Model file for the job. Use its own axes, mm. A direction names the side the tool comes from. Round coordinates to 2 decimals unless told otherwise and drop trailing zeros. Loops run counter-clockwise (first coordinate to the right, second up) from the corner with the lowest first, then second, coordinate; pieces in that order, holes last. Notation, with made-up numbers: (8, 19.25) -> (61, 19.25) arc R13 ccw to (61, 36.25) -> close; hole circle Ø11 at (69.25, -11). An arc over 180 degrees is marked (long way). Use a Markdown table: item, result.
from build123d import *

# Parameters (mm, degrees)
F1_DEPTH = 63.5
F0_W     = 25.4
F0_H     = 19.05
F2_DEPTH = 25.4
F3_DEPTH = 7.9375


with BuildPart() as f1:
    # F0 (on Front) → F1 (new body, symmetric)
    with BuildSketch(Plane.XZ):
        Polygon((41.275, -9.525), (41.275, 9.525), (22.225, 9.525), (-41.275, 9.525), (-41.275, -9.525), align=None)
    extrude(amount=F1_DEPTH, both=True)

    # F0 (on Front) → F2 (join, symmetric)
    with BuildSketch(Plane.XZ):
        with BuildLine():
            Line((22.225, 9.525), (41.275, 9.525))
            Line((41.275, 9.525), (41.275, 27.0002))
            ThreePointArc((41.275, 27.0002), (45.9246798487, 38.2255201513), (57.15, 42.8752))
            Line((57.15, 42.8752), (60.325, 42.8752))
            Line((60.325, 42.8752), (60.325, 61.9252))
            Line((60.325, 61.9252), (57.15, 61.9252))
            add(Edge.make_bspline(
                [(55.6374674655, 61.8924322349), (56.1423918101, 61.9048336292), (56.6465953403, 61.9157496607), (57.15, 61.9252)],
                knots=[110.2644548884, 110.2644548884, 110.2644548884, 110.2644548884, 111.5045361635, 111.5045361635, 111.5045361635, 111.5045361635], degree=3))
            ThreePointArc((55.6374674655, 61.8924322349), (31.9252024412, 51.1552245936), (22.225, 27.0002))
            Line((22.225, 27.0002), (22.225, 9.525))
        make_face()
        with Locations((73.025, 52.4002)):
            Rectangle(F0_W, F0_H)
    extrude(amount=F2_DEPTH, both=True)

    # F0 (on Front) → F3 (join, symmetric)
    with BuildSketch(Plane.XZ):
        with BuildLine():
            Line((-41.275, 9.525), (22.225, 9.525))
            Line((22.225, 9.525), (22.225, 27.0002))
            ThreePointArc((22.225, 27.0002), (31.9252024412, 51.1552245936), (55.6374674655, 61.8924322349))
            add(Edge.make_bspline(
                [(-41.275, 9.525), (-39.8543103668, 47.9433842004), (10.7410491974, 60.789735975), (55.6374674655, 61.8924322349)],
                knots=[0, 0, 0, 0, 110.2644548884, 110.2644548884, 110.2644548884, 110.2644548884], degree=3))
        make_face()
    extrude(amount=F3_DEPTH, both=True)

    # F0 (on Front) → F4 (revolve)
    with BuildSketch(Plane.XZ):
        Polygon((85.725, 61.9252), (85.725, 42.8752), (85.725, 38.1), (111.125, 38.1), (111.125, 66.675), (85.725, 66.675), align=None)
    revolve(axis=Axis((85.725, 0, 52.3875), (0, 0, 1)))


solid = f1.part
Q1. Drill centre lines: L1, parallel to Z at x = 17, y = -20 (3 decimals); L2, parallel to Y at x = -11, z = 38; L3, parallel to Y at x = 77.5, z = 48.5. Where is each one in solid material? Low to high. Write a range as from..to.
Results list:
| item | result |
|---|---|
| L1 | z = -9.525..9.525 |
| L2 | y = -7.94..7.94 |
| L3 | y = -25.4..25.4 |
Q2. Flat gauge pins, fed straight in: pin 1 (16.5 mm diameter, centred on x = 2.5, y = -47.5, fed in from +Z) (3 decimals); pin 2 (5 mm diameter, centred on y = 19.5, z = 54.5, fed in from +X); pin 3 (11 mm diameter, centred on y = -10, z = 3, fed in from +X) (3 decimals). Where does each tip first touch, or does it go through?
Results list:
| item | result |
|---|---|
| pin 1 | stops at z = 9.525 |
| pin 2 | stops at x = 104.6 |
| pin 3 | stops at x = 41.275 |
Q3. Band-saw the part on A-A, the plane y = -29. Give the cut face in (x, z) (3 decimals).
Results list:
| item | result |
|---|---|
| outline | (-41.275, -9.525) -> (41.275, -9.525) -> (41.275, 9.525) -> (-41.275, 9.525) -> close |
Q4. Pull direction X, two halves, no side cores. Call faces 1 (the face through (60, 2, 42.875)), 2 (the face through (60, -2, 61.925)), 3 (the face through (32.18, 16.55, 51.42)): released by +X, released by -X, zero draft, split by the parting line, or undercut.
Results list:
| item | result |
|---|---|
| face 1 | undercut |
| face 2 | zero draft |
| face 3 | released by -X |
Q5. Tool access for faces 4 (the face through (46, 25.4, 42)), 5 (the face through (45.8, -0.4, 38.1)), 6 (the face through (-4, 7.938, 30)), 7 (the face through (-4, -7.938, 30)), 8 (the face through (41.275, -1, 4)): list every direction of +Z, -Z, +X, -X, +Y, -Y with a clear straight run to the whole face (end or side of a thin tool).
Results list:
| item | result |
|---|---|
| face 4 | +Z, +X, -X, +Y |
| face 5 | -Z, +Y, -Y |
| face 6 | +Z, -X, +Y |
| face 7 | +Z, -X, -Y |
| face 8 | -Z, +X, +Y, -Y |
